Check sheet for the drawn part. Datum: minimum x, y, z corner. Units: mm. Coordinates: 2 decimals unless noted, no trailing zeros. Loops run counter-clockwise (first coordinate to the right, second up) from the corner with the lowest first, then second, coordinate; pieces in that order, holes last. Notation, with made-up numbers: M 45,-18 L 71,-18 A28 ccw 71,0 Z; hole C -35,89 d8. An arc over 180 degrees is marked long. Answer in a Markdown table with one row per item. Add a question column.
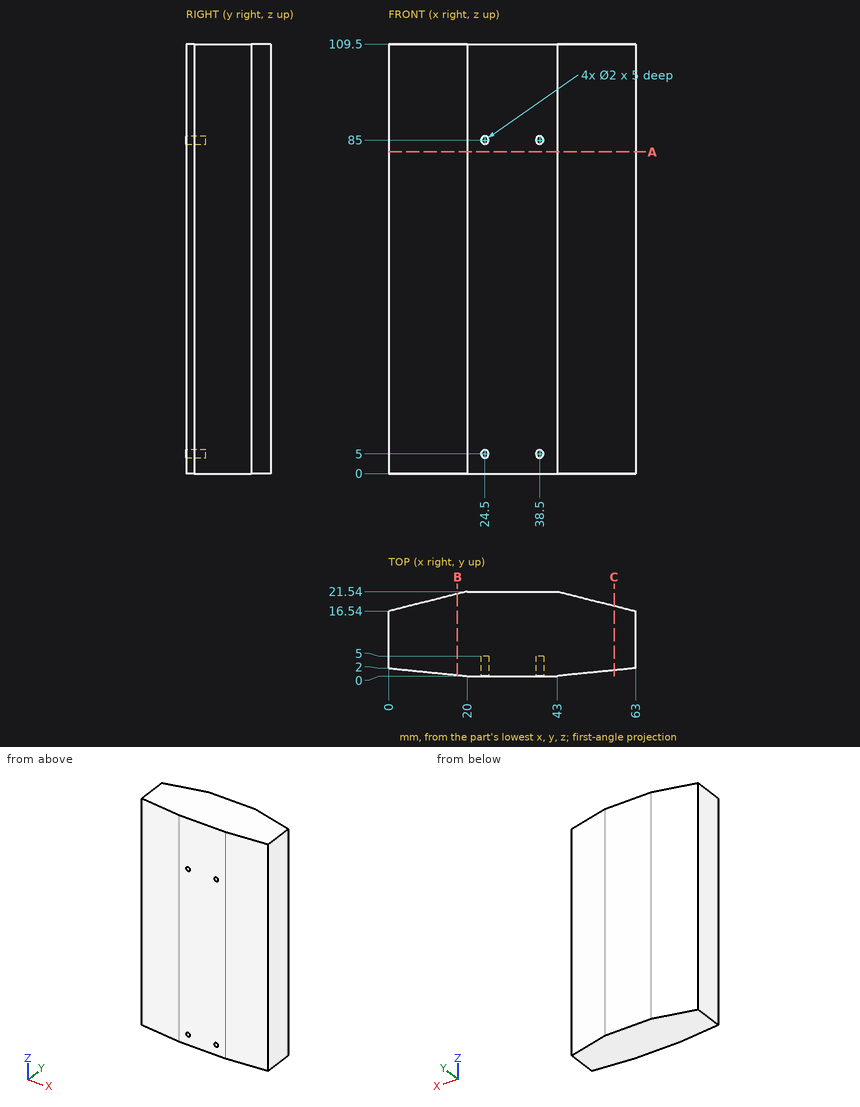
Q1. Cross-section at C-C (x = 57.5). Record the cut outline in (y, z) (3 decimals), plus the area to 3 significant figures.
Q2. Cross-section at B-B (x = 17.5). Record the cut outline in (y, z) (3 decimals).
Q3. Thickness scan on L1, parallel to X at y = 3.2, z = 85; L2, parallel to Z at x = 38.5, y = 4; L3, parallel to Y at x = 55, z = 57.5. Record the ranges inside material, lowest first.
Q4. Go/stop test with flat-tipped pins: pin 1 (1.5 mm diameter, centred on x = 12, z = 36, fed in from -Y) (3 decimals); pin 2 (1 mm diameter, centred on x = 38.5, z = 5, fed in from -Y). Record where each tip stops, or that it passes through.
Q5. Cross-section at A-A (z = 82). Record the cut outline in (x, y), plus the area to 3 significant figures.
Answer key:
| question | item | result |
|---|---|---|
| 1 | outline | M 1.45,0 L 17.915,0 L 17.915,109.5 L 1.45,109.5 Z |
| 1 | area | 1,800 mm^2 |
| 2 | outline | M 0.25,0 L 20.915,0 L 20.915,109.5 L 0.25,109.5 Z |
| 3 | L1 | 0 to 23.5, 25.5 to 37.5, 39.5 to 63 |
| 3 | L2 | 0 to 4, 6 to 84, 86 to 109.5 |
| 3 | L3 | 1.2 to 18.54 |
| 4 | pin 1 | y = 0.725 |
| 4 | pin 2 | y = 5 |
| 5 | outline | M 0,2 L 20,0 L 43,0 L 63,2 L 63,16.54 L 43,21.54 L 20,21.54 L 0,16.54 Z |
| 5 | area | 1,220 mm^2 |
